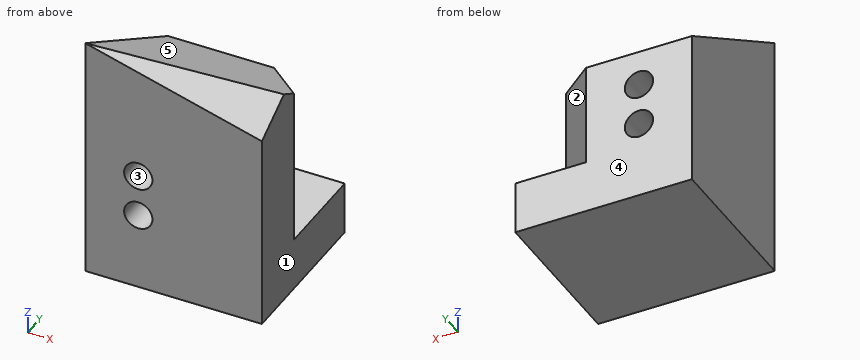
from build123d import *

# Parameters (mm, degrees)
SKETCH1_W           = 50
SKETCH1_H           = 45
BOSS_EXTRUDE1_DEPTH = 35
CUT_EXTRUDE1_DEPTH  = 51
CUT_EXTRUDE2_DEPTH  = 70
SKETCH20_R          = 4
CUT_EXTRUDE5_DEPTH  = 46
CUT_EXTRUDE6_DEPTH  = 56


with BuildPart() as part:
    # Sketch1 → Boss-Extrude1 (new body, symmetric)
    with BuildSketch(Plane.XY):
        with Locations((25, 22.5)):
            Rectangle(SKETCH1_W, SKETCH1_H)
    extrude(amount=BOSS_EXTRUDE1_DEPTH, both=True)

    # Sketch3 → Cut-Extrude1 (cut, through all)
    with BuildSketch(Plane(origin=(0, 0, 0), x_dir=(0, 0, -1), z_dir=(1, 0, 0))):
        Polygon((-35, 45), (-35, 0), (-9.019237886, 45), align=None)
    extrude(amount=CUT_EXTRUDE1_DEPTH, mode=Mode.SUBTRACT)

    # Sketch9 → Cut-Extrude2 (cut, along a direction that is not the sketch's normal)
    with BuildSketch(Plane(origin=(0, 15.155444566, 26.25), x_dir=(1, 0, 0), z_dir=(0, 0.5, 0.866025404))):
        Polygon((50, -17.5), (50, -3.643593539), (0, -17.5), align=None)
    extrude(amount=-CUT_EXTRUDE2_DEPTH, dir=(0, 0.866025404, 0.5), mode=Mode.SUBTRACT)

    # Sketch20 → Cut-Extrude5 (cut, through all)
    with BuildSketch(Plane(origin=(0, 0, 0), x_dir=(1, 0, 0), z_dir=(0, 1, 0))):
        with Locations((15, 13)):
            Circle(SKETCH20_R)
        with Locations((15, 1)):
            Circle(SKETCH20_R)
    extrude(amount=CUT_EXTRUDE5_DEPTH, mode=Mode.SUBTRACT)

    # Sketch23 → Cut-Extrude6 (cut, through all)
    with BuildSketch(Plane.XY.offset(-20)):
        Polygon((50, 45), (30, 45), (50, 17.320508076), align=None)
    extrude(amount=CUT_EXTRUDE6_DEPTH, mode=Mode.SUBTRACT)


solid = part.part
Can you work these out from the model? Positions are in its coordinate system, mm. Face numbers are marked on the shaded views. A direction names the side the tool comes from. Coordinates: 2 decimals unless noted, no trailing zeros. Loops run counter-clockwise (first coordinate to the right, second up) from the corner with the lowest first, then second, coordinate; pieces in that order, holes last. Notation, with made-up numbers: M 46,-37.5 L 66,-37.5 A13 cw 66,-29.5 Z; hole C 24.5,-8.5 d9. An arc over 180 degrees is marked long. Return JSON: item names as keys, results as strings. Group by question number.
Item 1: Imagine slicing it at A-A (z = -13). Please give me the cut outline in (x, y).
Item 2: Imagine slicing it at B-B (y = 7). Please give me the cut outline in (x, z).
Item 3: Imagine slicing it at C-C (x = 15). Please give me the cut outline in (y, z).
Item 4: If I drill on L1, parallel to X at y = 9, z = -1; L2, parallel to Z at x = 15, y = 9; L3, parallel to Z at x = 15, y = 30, over which ranges is the centre line in solid material (lowest first)? Write a range as from..to.
Item 5: Thinking about a two-plate mould opening in Z: for the marked faces 3, 4 and 5, which applies, released by +Z, released by -Z, zero draft, split by the parting line, or undercut?
Item 6: I'm going to push flat-ended pins straight in: pin 1 Ø2 at (x, y) = (18.5, 40) entering from +Z; pin 2 Ø12 at (y, z) = (27.5, 18) entering from -X; pin 3 Ø10 at (y, z) = (22.5, 23.5) entering from +X; pin 4 Ø4 at (y, z) = (25.5, -3) entering from +X. Where does each tip first touch, or does it pass through?
Item 7: On a 3-axis mill with a long thin cutter (end or side, diameter ignored), from which of +Z, -Z, +X, -X, +Y, -Y can I reach the whole of each face in a straight line? I mean the marked faces 1 and 2. Say none if no direction works.
Item 8: Imagine slicing it at D-D (z = 6). Please give me the cut outline in (x, y), and give its area (3 significant figures).
Verdict:
{
 "1": {"outline": "M 0,0 L 11,0 L 11,45 L 0,45 Z; M 19,0 L 50,0 L 50,17.32 L 30,45 L 19,45 Z"},
 "2": {"outline": "M 0,-35 L 50,-35 L 50,25.19 L 29.17,30.96 L 0,30.96 Z; hole C 15,-13 d8; hole C 15,-1 d8"},
 "3": {"outline": "M 0,-35 L 45,-35 L 45,-17 L 0,-17 Z; M 0,-9 L 45,-9 L 45,-5 L 0,-5 Z; M 0,3 L 45,3 L 45,9.02 L 3.6,32.92 L 0,30.84 Z"},
 "4": {"L1": "x = 0..11, 19..50", "L2": "z = -35..-17, -9..-5, 3..29.8", "L3": "z = -35..-17, -9..-5, 3..17.68"},
 "5": {"face 3": "undercut", "face 4": "zero draft", "face 5": "released by +Z"},
 "6": {"pin 1": "stops at z = 12.48", "pin 2": "stops at x = 0", "pin 3": "stops at x = 49.87", "pin 4": "stops at x = 45.53"},
 "7": {"face 1": "+Z, -Z, +X, +Y, -Y", "face 2": "+Z, +X, +Y"},
 "8": {"outline": "M 0,0 L 50,0 L 50,17.32 L 30,45 L 0,45 Z", "area": "1,970 mm^2"}
}
